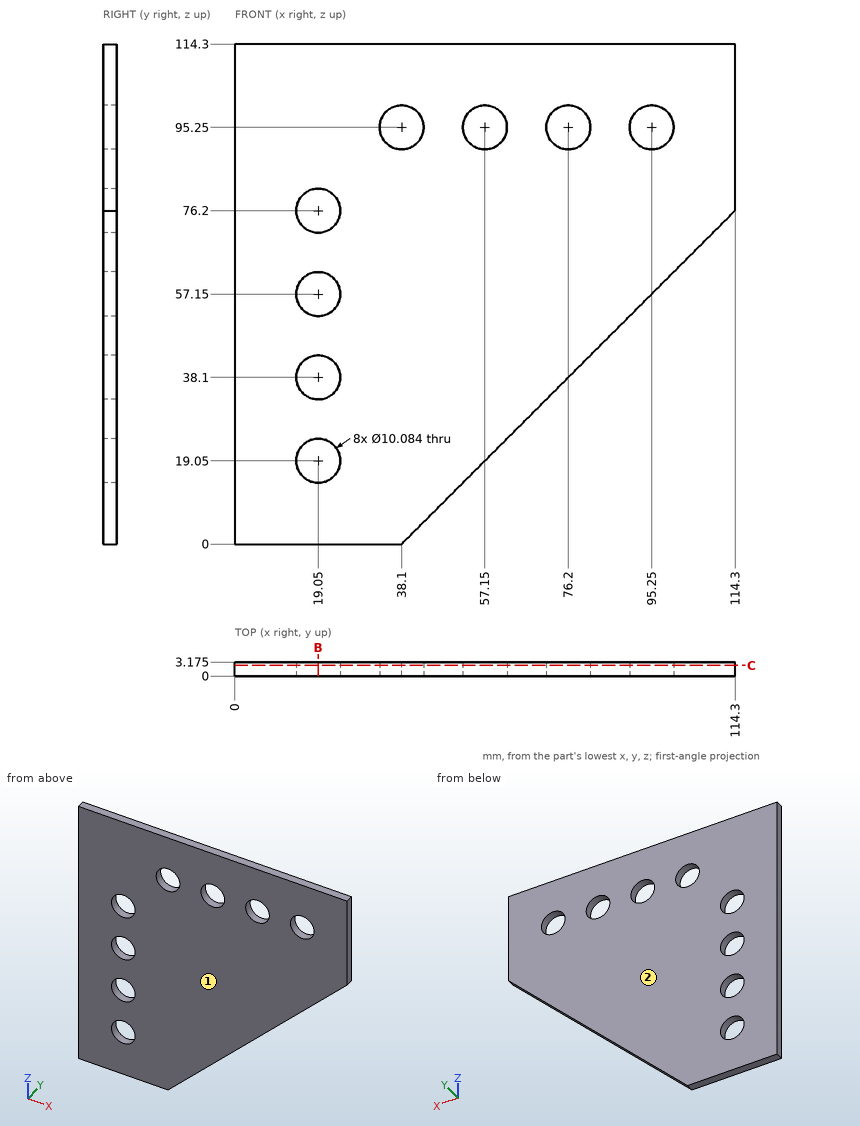
Design review of the part shown in the three views and the two pictorial views. Dimensions are in mm from the part's minimum x, y and z. Coordinates: 2 decimals unless noted, no trailing zeros. Order: outer loops, then holes, each group sorted by start corner. A loop starts at its lowest first (then second) coordinate and runs counter-clockwise, first axis right, second up.
Item 1: For line 1 (X direction, y = 2.5, z = 95.25); line 2 (Z direction, x = 19.05, y = 1.05); line 3 (Z direction, x = 38.1, y = 1.4), list the stretches that pass through material, from the lowest coordinate up.
Item 2: The part is to be moulded in two halves that separate along Y. For the marked faces 1 and 2, say which applies: pulls with the +Y half, pulls with the -Y half, needs draft (parallel to the pull), parting line crosses it, or undercut.
Item 3: For pin 1 Ø6 at (x, z) = (19.05, 19.05) entering from -Y, flat-tipped, find the tip position at first contact; note if it passes through.
Item 4: Take a section at B-B, the plane x = 19.05. Write out the cut boundary in (y, z) (1 decimal), then the cut area to 3 significant figures.
Item 5: Take a section at C-C, the plane y = 2.4. Count the separate pieces of the cut face and the enclosed holes in it, then the cut area to 3 significant figures.
The answers:
1. line 1: x = 0 to 33.06, 43.14 to 52.11, 62.19 to 71.16, 81.24 to 90.21, 100.29 to 114.3
1. line 2: z = 0 to 14.01, 24.09 to 33.06, 43.14 to 52.11, 62.19 to 71.16, 81.24 to 114.3
1. line 3: z = 0 to 90.21, 100.29 to 114.3
2. face 1: pulls with the -Y half
2. face 2: pulls with the +Y half
3. pin 1: passes through
4. outline: (0, 0) - (3.2, 0) - (3.2, 14) - (0, 14) - close; (0, 24.1) - (3.2, 24.1) - (3.2, 33.1) - (0, 33.1) - close; (0, 43.1) - (3.2, 43.1) - (3.2, 52.1) - (0, 52.1) - close; (0, 62.2) - (3.2, 62.2) - (3.2, 71.2) - (0, 71.2) - close; (0, 81.2) - (3.2, 81.2) - (3.2, 114.3) - (0, 114.3) - close
4. area: 235 mm2
5. separate pieces: 1
5. enclosed holes: 8
5. area: 9,520 mm2
